```python
from build123d import *

# Parameters (mm, degrees)
F0_W     = 609.6
F0_H     = 304.8
F1_DEPTH = 3.175
F2_W     = 76.2
F2_H     = 3.175
F3_DEPTH = 3.176
F4_W     = 3.175
F4_H     = 76.2
F4_H_2   = 73.025
F5_DEPTH = 3.176


with BuildPart() as f1:
    # F0 (on Top) → F1 (new body)
    with BuildSketch(Plane.XY):
        with Locations((84.824273, 1.423104)):
            Rectangle(F0_W, F0_H)
    extrude(amount=F1_DEPTH)

    # F2 (on face) → F3 (cut, through all)
    with BuildSketch(Plane.XY.offset(3.175)):
        with Locations((-181.875727, 152.235604)):
            Rectangle(F2_W, F2_H)
        with Locations((351.524273, 152.235604)):
            Rectangle(F2_W, F2_H)
        with Locations((-181.875727, -149.389396)):
            Rectangle(F2_W, F2_H)
        with Locations((351.524273, -149.389396)):
            Rectangle(F2_W, F2_H)
        with Locations((46.724273, 152.235604)):
            Rectangle(F2_W, F2_H)
        with Locations((122.924273, 152.235604)):
            Rectangle(F2_W, F2_H)
        with Locations((46.724273, -149.389396)):
            Rectangle(F2_W, F2_H)
        with Locations((122.924273, -149.389396)):
            Rectangle(F2_W, F2_H)
    extrude(amount=-F3_DEPTH, mode=Mode.SUBTRACT)

    # F4 (on face) → F5 (cut, through all)
    with BuildSketch(Plane.XY.offset(3.175)):
        with Locations((388.036773, 39.523104)):
            Rectangle(F4_W, F4_H)
        with Locations((388.036773, -111.289396)):
            Rectangle(F4_W, F4_H_2)
        with Locations((-218.388227, -111.289396)):
            Rectangle(F4_W, F4_H_2)
        with Locations((-218.388227, 39.523104)):
            Rectangle(F4_W, F4_H)
    extrude(amount=-F5_DEPTH, mode=Mode.SUBTRACT)


solid = f1.part
```
Check sheet for the modelled part. Datum: model origin and axes. Units: mm. Round coordinates to 2 decimals unless told otherwise and drop trailing zeros. Loops run counter-clockwise (first coordinate to the right, second up) from the corner with the lowest first, then second, coordinate; pieces in that order, holes last. Notation, with made-up numbers: M 49,-17 L 91,-17 A17 ccw 91,-9 Z; hole C -25.75,7 d7. An arc over 180 degrees is marked long. Answer as a JSON object with one key per item and string values.
1. Section check B-B (x = 36.5). Record the boundary of the cut face in (y, z) (3 decimals), plus the area to 3 significant figures.
Reply:
{"outline": "M -147.802,0 L 150.648,0 L 150.648,3.175 L -147.802,3.175 Z", "area": "948 mm²"}
2. Scan lines: line 1 (Y direction, x = 64.5, z = 1.25); line 2 (X direction, y = 68, z = 1.55). Record each from-to range of solid material in increasing order.
Reply:
{"line 1": "y = -147.8 to 150.65", "line 2": "x = -216.8 to 386.45"}
3. Gauge pin test, flat ends, axial feed: P1, Ø1.6, axis at y = -149, z = 1, coming from the -X side; P2, Ø1, axis at x = 89, z = 2, coming from the -Y side; P3, Ø1.5, axis at x = 135, z = 0.5, coming from the +Y side. Record the tip position at first contact, or that the pin passes through.
Reply:
{"P1": "stops at x = -143.78", "P2": "stops at y = -147.8", "P3": "stops at y = 150.65"}
